from build123d import *

# Parameters (mm, degrees)
F0_W          = 104.14
F0_H          = 135.89
F0_R          = 2.5
F0_R_2        = 1.5
F0_R_3        = 3.5
F1_DEPTH      = 2
F3_W          = 15
F3_H          = 15
F4_DEPTH      = 13
F4_DEPTH_BACK = 2
F5_W          = 18
F5_H          = 35.5
F6_DEPTH      = 17
F8_W          = 8
F8_H          = 3
F9_DEPTH      = 2


with BuildPart() as f1:
    # F0 (on Top) → F1 (new body)
    with BuildSketch(Plane.XY):
        Rectangle(F0_W, F0_H)
        with Locations((-44.07, -59.055)):
            Circle(F0_R, mode=Mode.SUBTRACT)
        with Locations((-48.26, -48.895)):
            Circle(F0_R_2, mode=Mode.SUBTRACT)
        with Locations((-44.07, -38.735)):
            Circle(F0_R, mode=Mode.SUBTRACT)
        with Locations((-44.07, -18.415)):
            Circle(F0_R, mode=Mode.SUBTRACT)
        with Locations((44.07, -59.055)):
            Circle(F0_R, mode=Mode.SUBTRACT)
        with Locations((48.26, -48.895)):
            Circle(F0_R_2, mode=Mode.SUBTRACT)
        with Locations((44.07, -38.735)):
            Circle(F0_R, mode=Mode.SUBTRACT)
        with Locations((44.07, -18.415)):
            Circle(F0_R, mode=Mode.SUBTRACT)
        with Locations((-44.07, 1.905)):
            Circle(F0_R, mode=Mode.SUBTRACT)
        with Locations((-44.07, 37.445)):
            Circle(F0_R_3, mode=Mode.SUBTRACT)
        with Locations((-48.26, 48.265)):
            Circle(F0_R_2, mode=Mode.SUBTRACT)
        with Locations((44.07, 1.905)):
            Circle(F0_R, mode=Mode.SUBTRACT)
        with Locations((48.26, 48.265)):
            Circle(F0_R_2, mode=Mode.SUBTRACT)
    extrude(amount=F1_DEPTH)

    # F3 (on offset) → F4 (join, two sides)
    with BuildSketch(Plane.XY.offset(2)) as f4_sk:
        with Locations((-39.74, 75.445)):
            Rectangle(F3_W, F3_H)
    extrude(amount=F4_DEPTH)
    extrude(f4_sk.sketch, amount=-F4_DEPTH_BACK)

    # F5 (on offset) → F6 (join)
    with BuildSketch(Plane.XY.offset(2)):
        with Locations((6.35, -50.195)):
            Rectangle(F5_W, F5_H)
    extrude(amount=F6_DEPTH)

    # F8 (on offset) → F9 (join)
    with BuildSketch(Plane.XZ.offset(67.945)):
        with Locations((6.35, 17.5)):
            Rectangle(F8_W, F8_H)
    extrude(amount=F9_DEPTH)


solid = f1.part
The listing builds one solid part. Answer for the finished solid, in the listing's coordinates (mm). A direction names the side the tool comes from. Give positions to 0.01 mm unless a question says otherwise; leave off trailing zeros. Loops run counter-clockwise (first coordinate to the right, second up) from the corner with the lowest first, then second, coordinate; pieces in that order, holes last.
Item 1: A cutting plane is placed at B-B (z = 7.5). Give the vertices of the cut face in (x, y) (3 decimals), then the cut area to 3 significant figures.
Derived:
outline: (-47.24, 67.945) - (-32.24, 67.945) - (-32.24, 82.945) - (-47.24, 82.945) - close; (-2.65, -67.945) - (15.35, -67.945) - (15.35, -32.445) - (-2.65, -32.445) - close
area: 864 mm2
Item 2: Each of these flat-tipped pins is pushed along its axis until it touches: pin 1 Ø0.6 at (y, z) = (-69, 18) entering from +X; pin 2 Ø1 at (x, y) = (8, -68.5) entering from -Z; pin 3 Ø5 at (x, y) = (48.26, -48.895) entering from +Z. Where does it stop, or does it pass through?
Derived:
pin 1: stops at x = 10.35
pin 2: stops at z = 16
pin 3: stops at z = 2
Item 3: A tool of negligible diameter and unlimited length cuts with its end or side. For faces 1 (the flat face through (-2.65, -50, 10)), 2 (the cylindrical face through (-42.455, 34.34, 0.986)), 3 (the flat face through (6, -32.445, 10)), from which of +Z, -Z, +X, -X, +Y, -Y can it reach the whole face along a straight path? Write none if from no direction.
Derived:
face 1: +Z, -X, +Y, -Y
face 2: +Z, -Z
face 3: +Z, +X, -X, +Y
Item 4: Find the intervals of material crossed by line 1 along Y through (x, z) = (44.07, 1.65) (3 decimals); line 2 along Y through (x, z) = (-44.07, 0.6) (3 decimals); line 3 along Y through (x, z) = (2, 5.75) (3 decimals), in increasing order.
Derived:
line 1: y = -67.945 to -61.555, -56.555 to -41.235, -36.235 to -20.915, -15.915 to -0.595, 4.405 to 67.945
line 2: y = -67.945 to -61.555, -56.555 to -41.235, -36.235 to -20.915, -15.915 to -0.595, 4.405 to 33.945, 40.945 to 82.945
line 3: y = -67.945 to -32.445
Item 5: A cutting plane is placed at A-A (x = 44.07). Give the vertices of the cut face in (y, z) (3 decimals), then the cut area to 3 significant figures.
Derived:
outline: (-67.945, 0) - (-61.555, 0) - (-61.555, 2) - (-67.945, 2) - close; (-56.555, 0) - (-41.235, 0) - (-41.235, 2) - (-56.555, 2) - close; (-36.235, 0) - (-20.915, 0) - (-20.915, 2) - (-36.235, 2) - close; (-15.915, 0) - (-0.595, 0) - (-0.595, 2) - (-15.915, 2) - close; (4.405, 0) - (67.945, 0) - (67.945, 2) - (4.405, 2) - close
area: 232 mm2
Item 6: A cutting plane is placed at C-C (x = -44.07). Give the vertices of the cut face in (y, z) (3 decimals), then the cut area to 3 significant figures.
Derived:
outline: (-67.945, 0) - (-61.555, 0) - (-61.555, 2) - (-67.945, 2) - close; (-56.555, 0) - (-41.235, 0) - (-41.235, 2) - (-56.555, 2) - close; (-36.235, 0) - (-20.915, 0) - (-20.915, 2) - (-36.235, 2) - close; (-15.915, 0) - (-0.595, 0) - (-0.595, 2) - (-15.915, 2) - close; (4.405, 0) - (33.945, 0) - (33.945, 2) - (4.405, 2) - close; (40.945, 0) - (82.945, 0) - (82.945, 15) - (67.945, 15) - (67.945, 2) - (40.945, 2) - close
area: 443 mm2
Item 7: Determine the mould class of faces 4 (the flat face through (6, -69.945, 18)), 5 (the cylindrical face through (49.69, 48.72, 0.99)), 6 (the cylindrical face through (46.38, -39.69, 0.99)), 7 (the flat face through (-1, 9, 0)) for opening direction Y: +Y half, -Y half, draft (parallel to the pull), parting line (faces both ways), or undercut.
Derived:
face 4: -Y half
face 5: undercut
face 6: undercut
face 7: draft
Item 8: A cutting plane is placed at D-D (y = 59). Give the vertices of the cut face in (x, z), then the cut area to 3 significant figures.
Derived:
outline: (-52.07, 0) - (52.07, 0) - (52.07, 2) - (-52.07, 2) - close
area: 208 mm2
